Work out the finished part from the listing and answer in its coordinate system (mm). A direction names the side the tool comes from. Coordinates: 2 decimals unless noted, no trailing zeros. Loops run counter-clockwise (first coordinate to the right, second up) from the corner with the lowest first, then second, coordinate; pieces in that order, holes last. Notation, with made-up numbers: (76, 26) - (104, 26) arc R29 ccw to (104, 47) - close; hole circle Ø11 at (58, -20). An arc over 180 degrees is marked (long way). Write each question's results on one line, items separated by ' | '. Start each with the question number.
Item 1: Section D-D, the plane y = -5 is taken. Write down the section's boundary in (x, z).
Item 2: A tool of negligible diameter and unlimited length cuts with its end or side. For faces 1 (the face through (0, -8.4, 1)), 2 (the face through (2.85, -7.79, 0.74)), 3 (the face through (-0.2, -9.2, -0.3)), from which of +Z, -Z, +X, -X, +Y, -Y can it reach the whole face along a straight path? Write none if from no direction.
Item 3: Each of these flat-tipped pins is pushed along its axis until it touches: pin 1 Ø1.5 at (y, z) = (-8, 0.5) entering from +X; pin 2 Ø1.5 at (y, z) = (-1.5, 1) entering from +X; pin 3 Ø0.7 at (y, z) = (-9, 1) entering from +X. Where does it stop, or does it pass through?
Item 4: Consider probe 1 along Y at (x, z) = (8.95, 0.65); probe 2 along X at (y, z) = (-0.25, -0.3); probe 3 along X at (y, z) = (7, 0.8). Determine where each line is inside the solid, lowest interval first. Write a range as [from, to].
Item 5: Section C-C, the plane x = -7.5 is taken. Write down the section's boundary in (y, z), plus the area to 3 significant figures.
Item 6: Section B-B, the plane y = -0.75 is taken. Write down the section's boundary in (x, z), plus the area to 3 significant figures.
Item 7: For a pull along X with two mould halves and no side action, classify faces 4 (the face through (-1.65, -5.6, 0.74)), 5 (the face through (-11.45, -9, 1)), 6 (the face through (0, 8.4, 1)), 7 (the face through (16.586, -7.717, -0.507)) as +X half, -X half, draft (parallel to the pull), parting line (faces both ways), or undercut.
Item 8: Section A-A, the plane z = 0.4 is taken. Write down the section's boundary in (x, y), plus the area to 3 significant figures.
from build123d import *

# Parameters (mm, degrees)
EXTRUDE_1_DEPTH     = 1.5
EXTRUDE_1_2_DEPTH   = 1.5
EXTRUDE_1_3_DEPTH   = 1.5
EXTRUDE_1_4_DEPTH   = 1.5
EXTRUDE_START       = 1
EXTRUDE_2_DEPTH     = 1
SKETCH_4_R          = 2.5
CUT_EXTRUDE_1_DEPTH = 21.501524334


with BuildPart() as part:
    # Sketch 2 → Extrude 1 (new body)
    with BuildSketch(Plane.XY):
        with BuildLine():
            Line((-1.93002849, -8.4), (1.93002849, -8.4))
            ThreePointArc((1.93002849, -8.4), (2.858869218, -7.770479287), (2.618260991, -6.674509804))
            ThreePointArc((2.618260991, -6.674509804), (1.659625246, -5.611633981), (0.87745098, -4.412930129))
            ThreePointArc((0.87745098, -4.412930129), (0, -3.892596448), (-0.87745098, -4.412930129))
            ThreePointArc((-0.87745098, -4.412930129), (-1.659625246, -5.611633981), (-2.618260991, -6.674509804))
            ThreePointArc((-2.618260991, -6.674509804), (-2.858869218, -7.770479287), (-1.93002849, -8.4))
        make_face()
    extrude(amount=EXTRUDE_1_DEPTH)



with BuildPart() as body_2:
    # Sketch 2 → Extrude 1 2 (new body)
    with BuildSketch(Plane.XY):
        with BuildLine():
            Line((1.93002849, 8.4), (-1.93002849, 8.4))
            ThreePointArc((-1.93002849, 8.4), (-2.858869218, 7.770479287), (-2.618260991, 6.674509804))
            ThreePointArc((-2.618260991, 6.674509804), (-1.659625246, 5.611633981), (-0.87745098, 4.412930129))
            ThreePointArc((-0.87745098, 4.412930129), (0, 3.892596448), (0.87745098, 4.412930129))
            ThreePointArc((0.87745098, 4.412930129), (1.659625246, 5.611633981), (2.618260991, 6.674509804))
            ThreePointArc((2.618260991, 6.674509804), (2.858869218, 7.770479287), (1.93002849, 8.4))
        make_face()
    extrude(amount=EXTRUDE_1_2_DEPTH)


with BuildPart() as body_3:
    # Sketch 2 → Extrude 1 3 (new body)
    with BuildSketch(Plane.XY):
        with BuildLine():
            Line((-11.45, -8.019351595), (-11.45, -7.809609465))
            ThreePointArc((-11.45, -7.809609465), (-8.95, 8.2), (-6.45, -7.809609465))
            Line((-6.45, -7.809609465), (-6.45, -8.019351595))
            Line((-6.45, -8.019351595), (-6.45, -9.2))
            Line((-6.45, -9.2), (-11.45, -9.2))
            Line((-11.45, -9.2), (-11.45, -8.019351595))
        make_face()
    extrude(amount=EXTRUDE_1_3_DEPTH)


with BuildPart() as body_4:
    # Sketch 2 → Extrude 1 4 (new body)
    with BuildSketch(Plane.XY):
        with BuildLine():
            Line((6.45, -8.019351595), (6.45, -7.809609465))
            ThreePointArc((6.45, -7.809609465), (8.95, 8.2), (11.45, -7.809609465))
            Line((11.45, -7.809609465), (11.45, -8.019351595))
            Line((11.45, -8.019351595), (11.45, -9.2))
            Line((11.45, -9.2), (6.45, -9.2))
            Line((6.45, -9.2), (6.45, -8.019351595))
        make_face()
    extrude(amount=EXTRUDE_1_4_DEPTH)


with BuildPart() as part_1:
    add(part.part)

    add(body_2.part)  # Extrude 2 merges body 2

    add(body_3.part)  # Extrude 2 merges body 3

    add(body_4.part)  # Extrude 2 merges body 4
    # Sketch 3 → Extrude 2 (add)
    with BuildSketch(Plane(origin=(0, 0, 0), x_dir=(-1, 0, 0), z_dir=(0, 0, -1)).offset(EXTRUDE_START)):
        with BuildLine():
            Line((-8.95, 9.2), (8.95, 9.2))
            ThreePointArc((8.95, 9.2), (15.455382387, 6.505382387), (18.15, 0))
            Line((18.15, 0), (18.15, -4))
            ThreePointArc((18.15, -4), (16.626955262, -7.676955262), (12.95, -9.2))
            Line((12.95, -9.2), (11.45, -9.2))
            Line((11.45, -9.2), (6.45, -9.2))
            Line((6.45, -9.2), (-6.45, -9.2))
            Line((-6.45, -9.2), (-11.45, -9.2))
            Line((-11.45, -9.2), (-12.95, -9.2))
            ThreePointArc((-12.95, -9.2), (-16.626955262, -7.676955262), (-18.15, -4))
            Line((-18.15, -4), (-18.15, 0))
            ThreePointArc((-18.15, 0), (-15.455382387, 6.505382387), (-8.95, 9.2))
        make_face()
    extrude(amount=-EXTRUDE_2_DEPTH)

    # Sketch 4 → Cut-Extrude 1 (cut, through all)
    with BuildSketch(Plane(origin=(0, 0, -1), x_dir=(-1, 0, 0), z_dir=(0, 0, -1))):
        with Locations((-8.95, 0)):
            Circle(SKETCH_4_R)
        with Locations((8.95, 0)):
            Circle(SKETCH_4_R)
    extrude(amount=-CUT_EXTRUDE_1_DEPTH, mode=Mode.SUBTRACT)


solid = part_1.part
Answer key:
1) outline: (-18.05, -1) - (18.05, -1) - (18.05, 0) - (15.45, 0) - (15.45, 1.5) - (2.45, 1.5) - (2.45, 0) - (1.23, 0) - (1.23, 1.5) - (-1.23, 1.5) - (-1.23, 0) - (-2.45, 0) - (-2.45, 1.5) - (-15.45, 1.5) - (-15.45, 0) - (-18.05, 0) - close
2) face 1: +Z, -Y | face 2: +Z | face 3: +Z, -Z, +X, -X, -Y
3) pin 1: stops at x = 16.85 | pin 2: stops at x = 17.12 | pin 3: stops at x = 11.45
4) probe 1: y = [-9.2, -2.5], [2.5, 8.2] | probe 2: x = [-18.15, -11.44], [-6.46, 6.46], [11.44, 18.15] | probe 3: x = [-13.22, -4.68], [-2.85, 2.85], [4.68, 13.22]
5) outline: (-9.2, -1) - (-2.04, -1) - (-2.04, 1.5) - (-9.2, 1.5) - close; (2.04, -1) - (9.2, -1) - (9.2, 0) - (8.07, 0) - (8.07, 1.5) - (2.04, 1.5) - close | area: 34.1 mm^2
6) outline: (-18.15, -1) - (-11.33, -1) - (-11.33, 1.5) - (-17.12, 1.5) - (-17.12, 0) - (-18.15, 0) - close; (-6.57, -1) - (6.57, -1) - (6.57, 1.5) - (0.78, 1.5) - (0.78, 0) - (-0.78, 0) - (-0.78, 1.5) - (-6.57, 1.5) - close; (11.33, -1) - (18.15, -1) - (18.15, 0) - (17.12, 0) - (17.12, 1.5) - (11.33, 1.5) - close | area: 61.4 mm^2
7) face 4: undercut | face 5: -X half | face 6: draft | face 7: +X half
8) outline: (-11.45, -9.2) - (-6.45, -9.2) - (-6.45, -7.81) arc R8.2 ccw (long way) to (-11.45, -7.81) - close; (-2.62, -6.67) arc R1 ccw to (-1.93, -8.4) - (1.93, -8.4) arc R1 ccw to (2.62, -6.67) arc R9.2 cw to (0.88, -4.41) arc R1 ccw to (-0.88, -4.41) arc R9.2 cw to start; (-2.62, 6.67) arc R9.2 cw to (-0.88, 4.41) arc R1 ccw to (0.88, 4.41) arc R9.2 cw to (2.62, 6.67) arc R1 ccw to (1.93, 8.4) - (-1.93, 8.4) arc R1 ccw to start; (6.45, -9.2) - (11.45, -9.2) - (11.45, -7.81) arc R8.2 ccw (long way) to (6.45, -7.81) - close; hole circle Ø5 at (-8.95, 0); hole circle Ø5 at (8.95, 0) | area: 430 mm^2
